The model under review builds one solid part; all positions refer to its coordinate system, in mm. Face numbers are marked on the shaded views. Round coordinates to 2 decimals unless told otherwise and drop trailing zeros. Loops run counter-clockwise (first coordinate to the right, second up) from the corner with the lowest first, then second, coordinate; pieces in that order, holes last. Notation, with made-up numbers: M 89.5,42.5 L 121.5,42.5 A29 cw 121.5,68.5 Z; hole C 42,52 d1. An arc over 180 degrees is marked long. Use a Markdown table: item, result. Add a question column.
```python
from build123d import *

# Parameters (mm, degrees)
BOSS_EXTRUDE1_DEPTH = 5


with BuildPart() as part:
    # Sketch1 → Boss-Extrude1 (new body)
    with BuildSketch(Plane(origin=(0, 0, 0), x_dir=(1, 0, 0), z_dir=(0, 1, 0))):
        with BuildLine():
            Line((0.885, 8.705129235), (0.785, 9.969141137))
            Line((0.785, 9.969141137), (0.5, 10.988630488))
            ThreePointArc((0.5, 10.988630488), (0, 11), (-0.5, 10.988630488))
            Line((-0.5, 10.988630488), (-0.785, 9.969141137))
            Line((-0.785, 9.969141137), (-0.885, 8.705129235))
            ThreePointArc((-0.885, 8.705129235), (-1.368801569, 8.64227298), (-1.848347855, 8.552549924))
            Line((-1.848347855, 8.552549924), (-2.334054665, 9.72379498))
            Line((-2.334054665, 9.72379498), (-2.920145308, 10.605317128))
            ThreePointArc((-2.920145308, 10.605317128), (-3.399186938, 10.461621679), (-3.871201824, 10.296300134))
            Line((-3.871201824, 10.296300134), (-3.827213396, 9.238638299))
            Line((-3.827213396, 9.238638299), (-3.531717889, 8.005589844))
            ThreePointArc((-3.531717889, 8.005589844), (-3.972416873, 7.796307087), (-4.400766544, 7.562787438))
            Line((-4.400766544, 7.562787438), (-5.224635797, 8.526616022))
            Line((-5.224635797, 8.526616022), (-6.054446447, 9.183881436))
            ThreePointArc((-6.054446447, 9.183881436), (-6.465637775, 8.899186938), (-6.863463441, 8.596096183))
            Line((-6.863463441, 8.596096183), (-6.494792479, 7.603793176))
            Line((-6.494792479, 7.603793176), (-5.832726624, 6.522407541))
            ThreePointArc((-5.832726624, 6.522407541), (-6.187184335, 6.187184335), (-6.522407541, 5.832726624))
            Line((-6.522407541, 5.832726624), (-7.603793176, 6.494792479))
            Line((-7.603793176, 6.494792479), (-8.596096183, 6.863463441))
            ThreePointArc((-8.596096183, 6.863463441), (-8.899186938, 6.465637775), (-9.183881436, 6.054446447))
            Line((-9.183881436, 6.054446447), (-8.526616022, 5.224635797))
            Line((-8.526616022, 5.224635797), (-7.562787438, 4.400766544))
            ThreePointArc((-7.562787438, 4.400766544), (-7.796307087, 3.972416873), (-8.005589844, 3.531717889))
            Line((-8.005589844, 3.531717889), (-9.238638299, 3.827213396))
            Line((-9.238638299, 3.827213396), (-10.296300134, 3.871201824))
            ThreePointArc((-10.296300134, 3.871201824), (-10.461621679, 3.399186938), (-10.605317128, 2.920145308))
            Line((-10.605317128, 2.920145308), (-9.72379498, 2.334054665))
            Line((-9.72379498, 2.334054665), (-8.552549924, 1.848347855))
            ThreePointArc((-8.552549924, 1.848347855), (-8.64227298, 1.368801569), (-8.705129235, 0.885))
            Line((-8.705129235, 0.885), (-9.969141137, 0.785))
            Line((-9.969141137, 0.785), (-10.988630488, 0.5))
            ThreePointArc((-10.988630488, 0.5), (-11, 0), (-10.988630488, -0.5))
            Line((-10.988630488, -0.5), (-9.969141137, -0.785))
            Line((-9.969141137, -0.785), (-8.705129235, -0.885))
            ThreePointArc((-8.705129235, -0.885), (-8.64227298, -1.368801569), (-8.552549924, -1.848347855))
            Line((-8.552549924, -1.848347855), (-9.72379498, -2.334054665))
            Line((-9.72379498, -2.334054665), (-10.605317128, -2.920145308))
            ThreePointArc((-10.605317128, -2.920145308), (-10.461621679, -3.399186938), (-10.296300134, -3.871201824))
            Line((-10.296300134, -3.871201824), (-9.238638299, -3.827213396))
            Line((-9.238638299, -3.827213396), (-8.005589844, -3.531717889))
            ThreePointArc((-8.005589844, -3.531717889), (-7.796307087, -3.972416873), (-7.562787438, -4.400766544))
            Line((-7.562787438, -4.400766544), (-8.526616022, -5.224635797))
            Line((-8.526616022, -5.224635797), (-9.183881436, -6.054446447))
            ThreePointArc((-9.183881436, -6.054446447), (-8.899186938, -6.465637775), (-8.596096183, -6.863463441))
            Line((-8.596096183, -6.863463441), (-7.603793176, -6.494792479))
            Line((-7.603793176, -6.494792479), (-6.522407541, -5.832726624))
            ThreePointArc((-6.522407541, -5.832726624), (-6.187184335, -6.187184335), (-5.832726624, -6.522407541))
            Line((-5.832726624, -6.522407541), (-6.494792479, -7.603793176))
            Line((-6.494792479, -7.603793176), (-6.863463441, -8.596096183))
            ThreePointArc((-6.863463441, -8.596096183), (-6.465637775, -8.899186938), (-6.054446447, -9.183881436))
            Line((-6.054446447, -9.183881436), (-5.224635797, -8.526616022))
            Line((-5.224635797, -8.526616022), (-4.400766544, -7.562787438))
            ThreePointArc((-4.400766544, -7.562787438), (-3.972416873, -7.796307087), (-3.531717889, -8.005589844))
            Line((-3.531717889, -8.005589844), (-3.827213396, -9.238638299))
            Line((-3.827213396, -9.238638299), (-3.871201824, -10.296300134))
            ThreePointArc((-3.871201824, -10.296300134), (-3.399186938, -10.461621679), (-2.920145308, -10.605317128))
            Line((-2.920145308, -10.605317128), (-2.334054665, -9.72379498))
            Line((-2.334054665, -9.72379498), (-1.848347855, -8.552549924))
            ThreePointArc((-1.848347855, -8.552549924), (-1.368801569, -8.64227298), (-0.885, -8.705129235))
            Line((-0.885, -8.705129235), (-0.785, -9.969141137))
            Line((-0.785, -9.969141137), (-0.5, -10.988630488))
            ThreePointArc((-0.5, -10.988630488), (0, -11), (0.5, -10.988630488))
            Line((0.5, -10.988630488), (0.785, -9.969141137))
            Line((0.785, -9.969141137), (0.885, -8.705129235))
            ThreePointArc((0.885, -8.705129235), (1.368801569, -8.64227298), (1.848347855, -8.552549924))
            Line((1.848347855, -8.552549924), (2.334054665, -9.72379498))
            Line((2.334054665, -9.72379498), (2.920145308, -10.605317128))
            ThreePointArc((2.920145308, -10.605317128), (3.399186938, -10.461621679), (3.871201824, -10.296300134))
            Line((3.871201824, -10.296300134), (3.827213396, -9.238638299))
            Line((3.827213396, -9.238638299), (3.531717889, -8.005589844))
            ThreePointArc((3.531717889, -8.005589844), (3.972416873, -7.796307087), (4.400766544, -7.562787438))
            Line((4.400766544, -7.562787438), (5.224635797, -8.526616022))
            Line((5.224635797, -8.526616022), (6.054446447, -9.183881436))
            ThreePointArc((6.054446447, -9.183881436), (6.465637775, -8.899186938), (6.863463441, -8.596096183))
            Line((6.863463441, -8.596096183), (6.494792479, -7.603793176))
            Line((6.494792479, -7.603793176), (5.832726624, -6.522407541))
            ThreePointArc((5.832726624, -6.522407541), (6.187184335, -6.187184335), (6.522407541, -5.832726624))
            Line((6.522407541, -5.832726624), (7.603793176, -6.494792479))
            Line((7.603793176, -6.494792479), (8.596096183, -6.863463441))
            ThreePointArc((8.596096183, -6.863463441), (8.899186938, -6.465637775), (9.183881436, -6.054446447))
            Line((9.183881436, -6.054446447), (8.526616022, -5.224635797))
            Line((8.526616022, -5.224635797), (7.562787438, -4.400766544))
            ThreePointArc((7.562787438, -4.400766544), (7.796307087, -3.972416873), (8.005589844, -3.531717889))
            Line((8.005589844, -3.531717889), (9.238638299, -3.827213396))
            Line((9.238638299, -3.827213396), (10.296300134, -3.871201824))
            ThreePointArc((10.296300134, -3.871201824), (10.461621679, -3.399186938), (10.605317128, -2.920145308))
            Line((10.605317128, -2.920145308), (9.72379498, -2.334054665))
            Line((9.72379498, -2.334054665), (8.552549924, -1.848347855))
            ThreePointArc((8.552549924, -1.848347855), (8.64227298, -1.368801569), (8.705129235, -0.885))
            Line((8.705129235, -0.885), (9.969141137, -0.785))
            Line((9.969141137, -0.785), (10.988630488, -0.5))
            ThreePointArc((10.988630488, -0.5), (11, 0), (10.988630488, 0.5))
            Line((10.988630488, 0.5), (9.969141137, 0.785))
            Line((9.969141137, 0.785), (8.705129235, 0.885))
            ThreePointArc((8.705129235, 0.885), (8.64227298, 1.368801569), (8.552549924, 1.848347855))
            Line((8.552549924, 1.848347855), (9.72379498, 2.334054665))
            Line((9.72379498, 2.334054665), (10.605317128, 2.920145308))
            ThreePointArc((10.605317128, 2.920145308), (10.461621679, 3.399186938), (10.296300134, 3.871201824))
            Line((10.296300134, 3.871201824), (9.238638299, 3.827213396))
            Line((9.238638299, 3.827213396), (8.005589844, 3.531717889))
            ThreePointArc((8.005589844, 3.531717889), (7.796307087, 3.972416873), (7.562787438, 4.400766544))
            Line((7.562787438, 4.400766544), (8.526616022, 5.224635797))
            Line((8.526616022, 5.224635797), (9.183881436, 6.054446447))
            ThreePointArc((9.183881436, 6.054446447), (8.899186938, 6.465637775), (8.596096183, 6.863463441))
            Line((8.596096183, 6.863463441), (7.603793176, 6.494792479))
            Line((7.603793176, 6.494792479), (6.522407541, 5.832726624))
            ThreePointArc((6.522407541, 5.832726624), (6.187184335, 6.187184335), (5.832726624, 6.522407541))
            Line((5.832726624, 6.522407541), (6.494792479, 7.603793176))
            Line((6.494792479, 7.603793176), (6.863463441, 8.596096183))
            ThreePointArc((6.863463441, 8.596096183), (6.465637775, 8.899186938), (6.054446447, 9.183881436))
            Line((6.054446447, 9.183881436), (5.224635797, 8.526616022))
            Line((5.224635797, 8.526616022), (4.400766544, 7.562787438))
            ThreePointArc((4.400766544, 7.562787438), (3.972416873, 7.796307087), (3.531717889, 8.005589844))
            Line((3.531717889, 8.005589844), (3.827213396, 9.238638299))
            Line((3.827213396, 9.238638299), (3.871201824, 10.296300134))
            ThreePointArc((3.871201824, 10.296300134), (3.399186938, 10.461621679), (2.920145308, 10.605317128))
            Line((2.920145308, 10.605317128), (2.334054665, 9.72379498))
            Line((2.334054665, 9.72379498), (1.848347855, 8.552549924))
            ThreePointArc((1.848347855, 8.552549924), (1.368801569, 8.64227298), (0.885, 8.705129235))
        make_face()
        with BuildLine():
            Line((1.5, 2), (1.5, -2))
            ThreePointArc((1.5, -2), (-2.5, 0), (1.5, 2))
        make_face(mode=Mode.SUBTRACT)
    extrude(amount=BOSS_EXTRUDE1_DEPTH)


solid = part.part
```
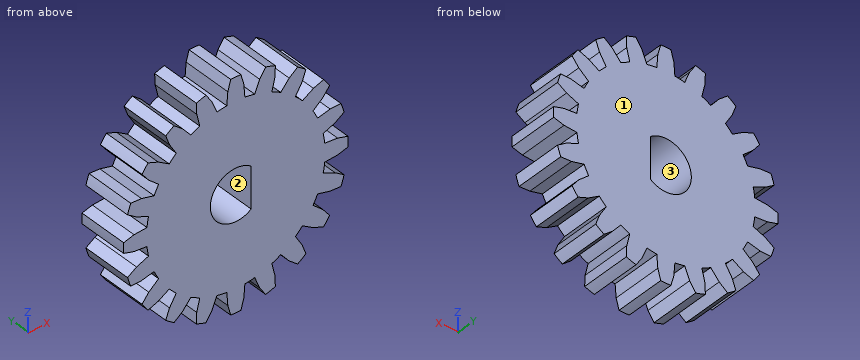
(1) To check wall thickness, follow probe 1 along Z at (x, y) = (9, 4.75); probe 2 along Z at (x, y) = (-9.5, 1.75); probe 3 along Z at (x, y) = (9.25, 4.3). State the ranges of each line that lie inside material, in increasing order.
(2) Draft analysis for pull direction X (two halves, no side actions). For the marked faces 1, 2 and 3, state which applies: released by +X, released by -X, zero draft, split by the parting line, or undercut.
(3) Insertion check: pin 1 Ø4 at (x, z) = (4, -8) entering from -Y; pin 2 Ø2 at (x, y) = (-4, 2) entering from -Z; pin 3 Ø2 at (x, y) = (-6.5, 1) entering from -Z; pin 4 Ø2 at (y, z) = (2, -3) entering from -X. Each pin has a flat end and moves straight along its axis. Give the tip position at first contact, or say it passes through.
(4) Consider section B-B, the plane z = 0. Give the boundary of the cut face in (x, y), then the cut area to 3 significant figures.
(5) Consider section A-A, the plane x = 0. Give the boundary of the cut face in (y, z).
Found:
| question | item | result |
|---|---|---|
| 1 | probe 1 | z = -6.32 to -5.82, -3.77 to -2.03, -0.86 to 0.86, 2.03 to 3.77, 5.82 to 6.32 |
| 1 | probe 2 | z = -3.84 to -2.24, -0.82 to 0.82, 2.24 to 3.84 |
| 1 | probe 3 | z = -3.83 to -2.14, -0.84 to 0.84, 2.14 to 3.83 |
| 2 | face 1 | zero draft |
| 2 | face 2 | undercut |
| 2 | face 3 | undercut |
| 3 | pin 1 | stops at y = 0 |
| 3 | pin 2 | stops at z = -10.58 |
| 3 | pin 3 | stops at z = -9.18 |
| 3 | pin 4 | stops at x = -10.61 |
| 4 | outline | M -11,0 L -2.5,0 L -2.5,5 L -11,5 Z; M 1.5,0 L 11,0 L 11,5 L 1.5,5 Z |
| 4 | area | 90.0 mm^2 |
| 5 | outline | M 0,-11 L 5,-11 L 5,-2.5 L 0,-2.5 Z; M 0,2.5 L 5,2.5 L 5,11 L 0,11 Z |
